Part model, mm, in its own coordinate system. A direction names the side the tool comes from. Round coordinates to 2 decimals unless told otherwise and drop trailing zeros. Order: outer loops, then holes, each group sorted by start corner. A loop starts at its lowest first (then second) coordinate and runs counter-clockwise, first axis right, second up. Notation, with made-up numbers: (12, 39.5) -> (48, 39.5) arc R15 cw to (48, 52.5) -> close; hole circle Ø1 at (-8, -4.5). An arc over 180 degrees is marked (long way). Return JSON: item names as keys, results as strings. Group by question number.
from build123d import *

# Parameters (mm, degrees)
F1_DEPTH = 12
F4_DEPTH = 12


with BuildPart() as f1:
    # F0 (on Front) → F1 (new body)
    with BuildSketch(Plane.XZ):
        Polygon((36, 0), (-36, 0), (-36, -20), (-24, -20), (-12, -40), (12, -40), (24, -20), (36, -20), align=None)
    extrude(amount=F1_DEPTH)

    # F3 (on offset) → F4 (join)
    with BuildSketch(Plane.YZ.offset(6)):
        Polygon((0, 0), (0, -20), (0, -30), (25, -15), (25, 0), align=None)
    extrude(amount=-F4_DEPTH)


solid = f1.part
(1) Tool access for faces 1 (the flat face through (-30, -6, -20)), 2 (the flat face through (-6, 12, -11)), 3 (the flat face through (6, 12, -11)): list every direction of +Z, -Z, +X, -X, +Y, -Y with a clear straight run to the whole face (end or side of a thin tool).
(2) Saw through at A-A, the plane y = -3.5. List the corners of the cut face in (x, z).
(3) Probe L1, parallel to Y at x = -33, z = -19.5; L2, parallel to X at y = 20.5, z = -7.5; L3, parallel to Z at x = -29.5, y = -0.5. List the from-to ranges inside material, lowest first. Write a range as [from, to].
(4) Pin check, flat tips, straight feed: P1, Ø3.5, axis at x = 27.5, y = -4, coming from the -Z side; P2, Ø7.5, axis at y = 14.5, z = -19.5, coming from the -X side; P3, Ø6, axis at x = -19.5, z = -7.5, coming from the +Y side; P4, Ø10, axis at x = -6.5, y = -4, coming from the +Z side. Stop position of each tip, or through.
(5) Saw through at D-D, the plane y = 1.5. List the corners of the cut face in (x, z).
(6) Saw through at B-B, the plane z = -13. List the corners of the cut face in (x, y).
(7) Saw through at C-C, the plane x = 25. List the corners of the cut face in (y, z).
Results are:
{
 "1": {"face 1": "-Z, -X, +Y, -Y", "face 2": "+Z, -Z, -X, +Y", "face 3": "+Z, -Z, +X, +Y"},
 "2": {"outline": "(-36, -20) -> (-24, -20) -> (-12, -40) -> (12, -40) -> (24, -20) -> (36, -20) -> (36, 0) -> (-36, 0) -> close"},
 "3": {"L1": "y = [-12, 0]", "L2": "x = [-6, 6]", "L3": "z = [-20, 0]"},
 "4": {"P1": "stops at z = -20", "P2": "stops at x = -6", "P3": "stops at y = 0", "P4": "stops at z = 0"},
 "5": {"outline": "(-6, -29.1) -> (6, -29.1) -> (6, 0) -> (-6, 0) -> close"},
 "6": {"outline": "(-36, -12) -> (36, -12) -> (36, 0) -> (6, 0) -> (6, 25) -> (-6, 25) -> (-6, 0) -> (-36, 0) -> close"},
 "7": {"outline": "(-12, -20) -> (0, -20) -> (0, 0) -> (-12, 0) -> close"}
}
